```python
from build123d import *

# Parameters (mm, degrees)
EXTRUDE_9_DEPTH     = 16
SKETCH_12_W         = 3.587626489
SKETCH_12_H         = 2.400728999
CUT_EXTRUDE_2_DEPTH = 16
SKETCH_17_W         = 2
SKETCH_17_H         = 16
EXTRUDE_15_DEPTH    = 16
SKETCH_18_R         = 1
EXTRUDE_16_DEPTH    = 16


with BuildPart() as part:
    # 草图10 → 凸台-拉伸9 (new body)
    with BuildSketch(Plane.XY):
        with BuildLine():
            Line((-8.422649731, 1), (9, 1))
            Line((9, 1), (16.587626489, 1))
            Line((16.587626489, 1), (16.587626489, -1))
            Line((16.587626489, -1), (9, -1))
            Line((9, -1), (-9, -1))
            ThreePointArc((-9, -1), (-9.5, -0.866025404), (-9.866025404, -0.5))
            Line((-9.866025404, -0.5), (-17.866025404, 13.356406461))
            ThreePointArc((-17.866025404, 13.356406461), (-17.5, 14.722431864), (-16.133974596, 14.356406461))
            Line((-16.133974596, 14.356406461), (-8.422649731, 1))
        make_face()
    extrude(amount=EXTRUDE_9_DEPTH)

    # 草图12 → 切除-拉伸2 (cut)
    with BuildSketch(Plane.XY.offset(16)):
        with Locations((14.793813245, -0.2003645)):
            Rectangle(SKETCH_12_W, SKETCH_12_H)
    extrude(amount=-CUT_EXTRUDE_2_DEPTH, mode=Mode.SUBTRACT)

    # 草图17 → 凸台-拉伸15 (add)
    with BuildSketch(Plane.XZ.offset(1)):
        with Locations((12, 8)):
            Rectangle(SKETCH_17_W, SKETCH_17_H)
    extrude(amount=-EXTRUDE_15_DEPTH)

    # 草图18 → 凸台-拉伸16 (add)
    with BuildSketch(Plane(origin=(0, 15, 0), x_dir=(1, 0, 0), z_dir=(0, 1, 0))):
        with Locations((12, 0)):
            Circle(SKETCH_18_R)
        with Locations((12, -16)):
            Circle(SKETCH_18_R)
    extrude(amount=-EXTRUDE_16_DEPTH)


solid = part.part
```
Geometry check sheet. Reference: the model listing, model coordinates, mm. A direction names the side the tool comes from. Round coordinates to 2 decimals unless told otherwise and drop trailing zeros. Write each loop counter-clockwise with the first axis right and the second up, starting at its lowest first coordinate (ties: lowest second). Pieces come first, ordered by that corner, then holes. Notation, with made-up numbers: (28, 81) - (66, 81) arc R18 cw to (66, 111) - close; hole circle Ø9 at (-11, -34.75). An arc over 180 degrees is marked (long way). Write each question's results on one line, items separated by ' | '.
(1) Sectioned sample at B-B, the plane y = 2.75. Enter the section's corners in (x, z).
Computed:
outline: (-11.74, 0) - (-9.43, 0) - (-9.43, 16) - (-11.74, 16) - close; (11, 0) arc R1 ccw to (13, 0) - (13, 16) arc R1 ccw to (11, 16) - close
(2) Sectioned sample at D-D, the plane x = -17. Enter the section's corners in (y, z), plus the area to 3 significant figures.
Computed:
outline: (11.86, 0) - (14.86, 0) - (14.86, 16) - (11.86, 16) - close | area: 48.0 mm^2
(3) Draft check along X on faces 6 (the face through (11, 8, 8)), 7 (the face through (12, 7, 17)), 8 (the face through (12, 15, 8)). Enter one of: pulls with the +X half, pulls with the -X half, needs draft (parallel to the pull), parting line crosses it, or undercut.
Computed:
face 6: undercut | face 7: parting line crosses it | face 8: needs draft
(4) Thickness scan on probe 1 along Y at (x, z) = (-6.5, 15.5); probe 2 along X at (y, z) = (3.5, 14.75); probe 3 along X at (y, z) = (5.75, 2.25). Record the ranges inside material, lowest first. Write a range as from..to.
Computed:
probe 1: y = -1..1 | probe 2: x = -12.18..-9.87, 11..13 | probe 3: x = -13.47..-11.17, 11..13
(5) Sectioned sample at C-C, the plane x = -3.5. Enter the section's corners in (y, z).
Computed:
outline: (-1, 0) - (1, 0) - (1, 16) - (-1, 16) - close
(6) Sectioned sample at A-A, the plane z = 13. Enter the section's corners in (x, y).
Computed:
outline: (-17.87, 13.36) - (-9.87, -0.5) arc R1 ccw to (-9, -1) - (13, -1) - (13, 15) - (11, 15) - (11, 1) - (-8.42, 1) - (-16.13, 14.36) arc R1 ccw to start
(7) Set-up check for faces 1 (the face through (-5.6, 0.5, 0)), 2 (the face through (2, -1, 8)), 3 (the face through (-17.52, 14.71, 7.89)), 4 (the face through (-5.6, 0.5, 16)), 5 (the face through (-12.33, 7.77, 7.89)): record each of +Z, -Z, +X, -X, +Y, -Y from which the full face is reachable in a straight line by a thin tool's end or side.
Computed:
face 1: -Z, -X, +Y, -Y | face 2: +Z, -Z, +X, -X, -Y | face 3: +Z, -Z | face 4: +Z, -X, +Y, -Y | face 5: +Z, -Z, +Y
(8) Depth check by flat-ended pin: pin 1 Ø2 at (y, z) = (5.5, 5) entering from -X; pin 2 Ø5 at (x, y) = (-10, 7) entering from +Z; pin 3 Ø7 at (y, z) = (7.5, 10) entering from -X. Enter the tip coordinate at first touch or a pass-through.
Computed:
pin 1: stops at x = -13.91 | pin 2: stops at z = 16 | pin 3: stops at x = -16.51
